Verification items for the finished model (mm, model axes). A direction names the side the tool comes from. Round coordinates to 2 decimals unless told otherwise and drop trailing zeros. Order: outer loops, then holes, each group sorted by start corner. A loop starts at its lowest first (then second) coordinate and runs counter-clockwise, first axis right, second up. Notation, with made-up numbers: (48, 8) -> (93, 8) arc R28 ccw to (93, 46) -> close; hole circle Ø7 at (65.5, 25.5). An arc over 180 degrees is marked (long way). Return JSON: item names as keys, results as strings. Group by question number.
Item 1: Access from +Z, -Z, +X, -X, +Y, -Y to the whole of each face (thin tool, end or side, straight path). Record for faces 1 (the cylindrical face through (-91.388, 11.923, -3.755)), 2 (the cylindrical face through (71.779, -3.584, -2.285)), 3 (the cylindrical face through (1.23, 23.07, 44.36)).
Item 2: Draft check along Z on faces 4 (the flat face through (-100, -5.2, -0.2)), 5 (the cylindrical face through (91.612, 11.923, -3.755)), 6 (the cylindrical face through (-71, 2.285, 3.584)). Enter one of: pulls with the +Z half, pulls with the -Z half, needs draft (parallel to the pull), parting line crosses it, or undercut.
Item 3: Sectioned sample at A-A on x = 17. Record the cut outline in (y, z).
Item 4: Depth check by flat-ended pin: pin 1 Ø4 at (x, y) = (-62.5, 33) entering from +Z; pin 2 Ø6 at (y, z) = (-0.5, -28.5) entering from -X; pin 3 Ø10 at (x, y) = (44, 26.5) entering from +Z. Enter the tip coordinate at first touch or a pass-through.
Item 5: Scan lines: probe 1 along Y at (x, z) = (65.5, 0); probe 2 along Y at (x, z) = (-84, 0). Record each from-to range of solid material in increasing order. Write a range as from..to.
Item 6: Sectioned sample at B-B on x = -58. Record the cut outline in (y, z), plus the area to 3 significant figures.
```python
from build123d import *

# Parameters (mm, degrees)
CHAMFER1_SIZE                = 0.5
CHAMFER2_SIZE                = 3
CHAMFER2_SIZE2               = 3.300188603
CHAMFER3_SIZE                = 3
CHAMFER3_SIZE2               = 3.300188603
CHAMFER4_SIZE                = 0.5
M10_TAPPED_HOLE2_D           = 8.5
M10_TAPPED_HOLE2_DEPTH       = 56.446342369
M10_TAPPED_HOLE2_CSINK_D     = 10.05
M10_TAPPED_HOLE2_CSINK_ANGLE = 90
M10_TAPPED_HOLE2_TIP         = 2.553657631


with BuildPart() as part:
    # Sketch1 → Revolve1 (revolve)
    with BuildSketch(Plane.XY):
        Polygon((-100, 0), (-100, 12.5), (-83.5, 12.5), (-80.219175118, 50), (80.219175118, 50), (83.5, 12.5), (100, 12.5), (100, 0), align=None)
    revolve(axis=Axis((100, 0, 0), (-1, 0, 0)))

    # Chamfer1
    chamfer1_edges = [part.edges().sort_by_distance(p)[0] for p in [
        (-100, -12.5, 0),
    ]]
    chamfer(chamfer1_edges, length=CHAMFER1_SIZE)

    # Chamfer2
    chamfer2_edges = [part.edges().sort_by_distance(p)[0] for p in [
        (-80.219175118, -50, 0),
    ]]
    chamfer2_side = [part.faces().sort_by_distance(p)[0] for p in [
        (-81.859587559, -31.25, 0),
    ]]
    chamfer(chamfer2_edges, length=CHAMFER2_SIZE, length2=CHAMFER2_SIZE2, reference=chamfer2_side[0])

    # Chamfer3
    chamfer3_edges = [part.edges().sort_by_distance(p)[0] for p in [
        (80.219175118, -50, 0),
    ]]
    chamfer3_side = [part.faces().sort_by_distance(p)[0] for p in [
        (1.650094301, -50, 0),
    ]]
    chamfer(chamfer3_edges, length=CHAMFER3_SIZE, length2=CHAMFER3_SIZE2, reference=chamfer3_side[0])

    # Chamfer4
    chamfer4_edges = [part.edges().sort_by_distance(p)[0] for p in [
        (100, -12.5, 0),
    ]]
    chamfer(chamfer4_edges, length=CHAMFER4_SIZE)

    # Sketch5 → M10 Tapped Hole1 (revolve, cut)
    with BuildSketch(Plane(origin=(100, 0, 0), x_dir=(0, 0, -1), z_dir=(0, 1, 0))):
        Polygon((0, 0), (0, 59), (4.25, 56.446342369), (4.25, 0.775), (5.025, 0), align=None)
    revolve(axis=Axis((106.35, 0, 0), (-1, 0, 0)), mode=Mode.SUBTRACT)

    # M10 Tapped Hole2
    with Locations(Plane(origin=(-100, 0, 0), x_dir=(0, -1, 0), z_dir=(-1, 0, 0))):
        with Locations((0, 0)):
            CounterSinkHole(M10_TAPPED_HOLE2_D / 2, M10_TAPPED_HOLE2_CSINK_D / 2, depth=M10_TAPPED_HOLE2_DEPTH, counter_sink_angle=M10_TAPPED_HOLE2_CSINK_ANGLE)
            with Locations((0, 0, -(M10_TAPPED_HOLE2_DEPTH + M10_TAPPED_HOLE2_TIP / 2))):  # 118° drill point
                Cone(0, M10_TAPPED_HOLE2_D / 2, M10_TAPPED_HOLE2_TIP, mode=Mode.SUBTRACT)


solid = part.part
```
Recorded:
{
 "1": {"face 1": "-X", "face 2": "+X", "face 3": "+X, -X"},
 "2": {"face 4": "needs draft", "face 5": "parting line crosses it", "face 6": "undercut"},
 "3": {"outline": "circle Ø100 at (0, 0)"},
 "4": {"pin 1": "z = 39.23", "pin 2": "x = -82.36", "pin 3": "z = 45.14"},
 "5": {"probe 1": "-50..-4.25, 4.25..50", "probe 2": "-12.5..-4.25, 4.25..12.5"},
 "6": {"outline": "circle Ø100 at (0, 0); hole circle Ø8.5 at (0, 0)", "area": "7,800 mm²"}
}
